Design review of the part built by this model. Coordinates are the model's own, in mm. Give positions to 0.01 mm unless a question says otherwise; leave off trailing zeros. Order: outer loops, then holes, each group sorted by start corner. A loop starts at its lowest first (then second) coordinate and runs counter-clockwise, first axis right, second up. Notation, with made-up numbers: M -13.5,2 L 28.5,2 A4 ccw 28.5,7 Z; hole C 9,76 d10. An arc over 180 degrees is marked long. Answer as a JSON object with one key per item and string values.
from build123d import *

# Parameters (mm, degrees)
F0_R     = 22.225
F0_R_2   = 19.75
F1_DEPTH = 446.405
F3_DEPTH = 63.5
F4_W     = 7.893423
F4_H     = 2.54
F4_W_2   = 2.54
F4_H_2   = 8.828171
F5_DEPTH = 2.54


with BuildPart() as f1:
    # F0 (on Front) → F1 (new body)
    with BuildSketch(Plane.XZ):
        Circle(F0_R)
        Circle(F0_R_2, mode=Mode.SUBTRACT)
    extrude(amount=F1_DEPTH)

    # F2 (on Right) → F3 (cut, symmetric)
    with BuildSketch(Plane.YZ):
        with BuildLine():
            ThreePointArc((-38.1, 0), (-39.959872, 4.490128), (-44.45, 6.35))
            Line((-44.45, 6.35), (-211.455, 6.35))
            ThreePointArc((-211.455, 6.35), (-215.945128, 4.490128), (-217.805, 0))
            ThreePointArc((-217.805, 0), (-215.945128, -4.490128), (-211.455, -6.35))
            Line((-211.455, -6.35), (-44.45, -6.35))
            ThreePointArc((-44.45, -6.35), (-39.959872, -4.490128), (-38.1, 0))
        make_face()
        with BuildLine():
            Line((-236.855, 6.35), (-403.86, 6.35))
            ThreePointArc((-403.86, 6.35), (-408.350128, 4.490128), (-410.21, 0))
            ThreePointArc((-410.21, 0), (-408.350128, -4.490128), (-403.86, -6.35))
            Line((-403.86, -6.35), (-236.855, -6.35))
            ThreePointArc((-236.855, -6.35), (-232.364872, -4.490128), (-230.505, 0))
            ThreePointArc((-230.505, 0), (-232.364872, 4.490128), (-236.855, 6.35))
        make_face()
    extrude(amount=F3_DEPTH, both=True, mode=Mode.SUBTRACT)

    # F4 (on face) → F5 (cut)
    with BuildSketch(Plane.XZ.offset(446.405)):
        with Locations((22.911058, -1.27)):
            Rectangle(F4_W, F4_H)
        with Locations((1.27, 24.07)):
            Rectangle(F4_W_2, F4_H_2)
    extrude(amount=-F5_DEPTH, mode=Mode.SUBTRACT)


solid = f1.part
(1) We need section B-B (x = 11). Write out the cut boundary in (y, z) (3 decimals), plus the area to 3 significant figures.
Checked values:
{"outline": "M -446.405,-19.312 L 0,-19.312 L 0,-16.403 L -446.405,-16.403 Z; M -446.405,16.403 L 0,16.403 L 0,19.312 L -446.405,19.312 Z", "area": "2,600 mm^2"}
(2) Draft analysis for pull direction Z (two halves, no side actions). For faces 1 (the flat face through (0, 0, 20)), 2 (the cylindrical face through (21.199, -220.078, 6.676)), 3 (the cylindrical face through (-4.28, -220.08, -19.28)), state which applies: +Z half, -Z half, draft (parallel to the pull), parting line (faces both ways), or undercut.
Checked values:
{"face 1": "draft", "face 2": "parting line", "face 3": "undercut"}
(3) To check wall thickness, follow L1, parallel to Z at x = 0, y = -252 (3 decimals); L2, parallel to Z at x = -13, y = -182; L3, parallel to X at y = -101.5, z = -17.5. State the ranges of each line that lie inside material, in increasing order. Write a range as from..to.
Checked values:
{"L1": "z = -22.225..-19.75, 19.75..22.225", "L2": "z = -18.03..-14.87, 14.87..18.03", "L3": "x = -13.7..-9.15, 9.15..13.7"}
(4) We need section A-A (y = -262.5). Write out the cut boundary in (x, z) (3 decimals), plus the area to 3 significant figures.
Checked values:
{"outline": "M -21.299,-6.35 A22.225 ccw 21.299,-6.35 L 18.701,-6.35 A19.75 cw -18.701,-6.35 Z; M -21.299,6.35 L -18.701,6.35 A19.75 cw 18.701,6.35 L 21.299,6.35 A22.225 ccw Z", "area": "263 mm^2"}
(5) Insertion check: pin 1 (2 mm diameter, centred on x = -19.5, y = -341.5, fed in from +Z); pin 2 (0.8 mm diameter, centred on x = -20, y = -328, fed in from -Z); pin 3 (8 mm diameter, centred on y = -306, z = -2.5, fed in from +X). Each pin has a flat end and moves straight along its axis. Give the tip position at first contact, or say it passes through.
Checked values:
{"pin 1": "stops at z = 12.32", "pin 2": "stops at z = -10.48", "pin 3": "stops at x = 21.3"}
